Can you work these out from the model? Positions are in its coordinate system, mm. Face numbers are marked on the shaded views. A direction names the side the tool comes from. Round coordinates to 2 decimals unless told otherwise and drop trailing zeros. Write each loop counter-clockwise with the first axis right and the second up, starting at its lowest first coordinate (ties: lowest second). Pieces come first, ordered by that corner, then holes. Notation, with made-up numbers: (12, 70.25) -> (21, 70.25) arc R25 cw to (21, 104.25) -> close; hole circle Ø3 at (55, 3). An arc over 180 degrees is marked (long way). Use CSV: the item, a comma, the result in double quotes.
```python
from build123d import *

# Parameters (mm, degrees)
BOX009_W     = 45.5
BOX009_H     = 44
BOX009_DEPTH = 16
BOX018_W     = 54
BOX018_H     = 4.25
BOX018_DEPTH = 30.25
BOX027_W     = 4.25
BOX027_H     = 4.25
BOX027_DEPTH = 90.75
BOX013_W     = 4.25
BOX013_H     = 36.1
BOX013_DEPTH = 30.25


with BuildPart() as cable_exclusion_zone:
    # Box009 → Box009 (new body)
    with BuildSketch(Plane(origin=(126, 0, 7.125), x_dir=(-1, 0, 0), z_dir=(0, 0, 1))):
        with Locations((22.75, 22)):
            Rectangle(BOX009_W, BOX009_H)
    extrude(amount=BOX009_DEPTH)


with BuildPart() as cube001:
    # Box018 → Box018 (new body)
    with BuildSketch(Plane(origin=(72, -4.25, 0), x_dir=(1, 0, 0), z_dir=(0, 0, 1))):
        with Locations((27, 2.125)):
            Rectangle(BOX018_W, BOX018_H)
    extrude(amount=BOX018_DEPTH)


with BuildPart() as base_support001:
    # Box027 → Box027 (new body)
    with BuildSketch(Plane(origin=(126, 0, -30.25), x_dir=(-1, 0, 0), z_dir=(0, 0, 1))):
        with Locations((2.125, 2.125)):
            Rectangle(BOX027_W, BOX027_H)
    extrude(amount=BOX027_DEPTH)


with BuildPart() as fusion005:
    # Fusion005 base: copy of base_support001
    add(base_support001.part)

    # Fusion005: union Cube001
    add(cube001.part)


with BuildPart() as base_support:
    # Box013 → Box013 (new body)
    with BuildSketch(Plane(origin=(126, -4.25, 0), x_dir=(-1, 0, 0), z_dir=(0, 0, 1))):
        with Locations((2.125, 18.05)):
            Rectangle(BOX013_W, BOX013_H)
    extrude(amount=BOX013_DEPTH)


with BuildPart() as cut004:
    # Fusion006 base: copy of base_support001
    add(base_support001.part)

    # Fusion006: union Cube001, Fusion005, base_support
    add(cube001.part)
    add(fusion005.part)
    add(base_support.part)

    # Cut004: cut cable_exclusion_zone
    add(cable_exclusion_zone.part, mode=Mode.SUBTRACT)


solid = cut004.part
```
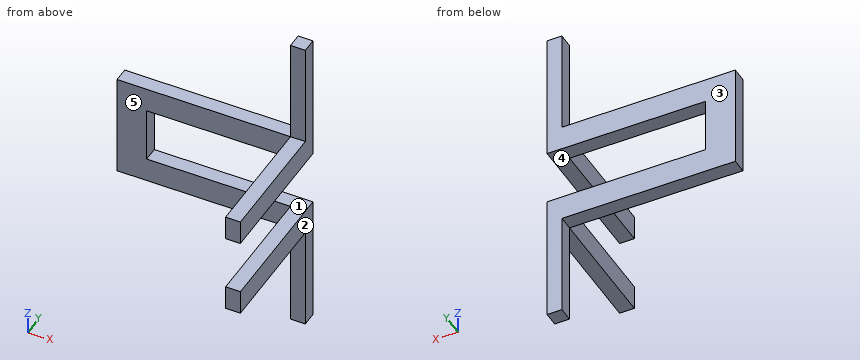
Q1. Suppose I cut it at C-C (z = 6). Write out the boundary of the cut face in (x, y).
Resolved:
outline,"(72, -4.25) -> (121.75, -4.25) -> (121.75, -40.35) -> (126, -40.35) -> (126, 0) -> (72, 0) -> close"
Q2. On a 3-axis mill with a long thin cutter (end or side, diameter ignored), from which of +Z, -Z, +X, -X, +Y, -Y can I reach the whole of each face in a straight line? I mean the marked faces 3, 4 and 5. Say none if no direction works.
Resolved:
face 3,"+Z, -Z, +X, -X, +Y"
face 4,"+X, +Y, -Y"
face 5,"+Z, -Z, -X, -Y"
Q3. If we mould it in two halves opening along Z, with no side actions, what happens to the marked faces 1 and 2? For each: released by +Z, released by -Z, zero draft, split by the parting line, or undercut.
Resolved:
face 1,"undercut"
face 2,"zero draft"
Q4. Suppose I cut it at B-B (x = 95.5). Write out the boundary of the cut face in (y, z) (3 decimals).
Resolved:
outline,"(-4.25, 0) -> (0, 0) -> (0, 7.125) -> (-4.25, 7.125) -> close; (-4.25, 23.125) -> (0, 23.125) -> (0, 30.25) -> (-4.25, 30.25) -> close"
Q5. Will these pins go through, and if not, where does the flat tip stop? P1, Ø3.5, axis at x = 124.5, z = -12.5, coming from the -Y side; P2, Ø1.3, axis at x = 88.5, y = -2.5, coming from the -Z side; P3, Ø1, axis at x = 98.5, z = 22, coming from the -Y side; P4, Ø3.5, axis at y = -1.5, z = 17.5, coming from the +X side.
Resolved:
P1,"stops at y = -4.25"
P2,"stops at z = 0"
P3,"passes through"
P4,"stops at x = 80.5"
Q6. Suppose I cut it at A-A (y = -31). Write out the boundary of the cut face in (x, z) (3 decimals).
Resolved:
outline,"(121.75, 0) -> (126, 0) -> (126, 7.125) -> (121.75, 7.125) -> close; (121.75, 23.125) -> (126, 23.125) -> (126, 30.25) -> (121.75, 30.25) -> close"
Q7. Please list where these lines run through material, in increasing order: probe 1 along Z at (x, y) = (123.5, -7) (3 decimals); probe 2 along X at (y, z) = (-36, 30); probe 3 along Y at (x, z) = (78.5, 23.5).
Resolved:
probe 1,"z = 0 to 7.125, 23.125 to 30.25"
probe 2,"x = 121.75 to 126"
probe 3,"y = -4.25 to 0"
Q8. Suppose I cut it at D-D (y = -3). Write out the boundary of the cut face in (x, z) (3 decimals), and give its area (3 significant figures).
Resolved:
outline,"(72, 0) -> (121.75, 0) -> (121.75, -30.25) -> (126, -30.25) -> (126, 7.125) -> (80.5, 7.125) -> (80.5, 23.125) -> (126, 23.125) -> (126, 60.5) -> (121.75, 60.5) -> (121.75, 30.25) -> (72, 30.25) -> close"
area,"1,160 mm^2"
